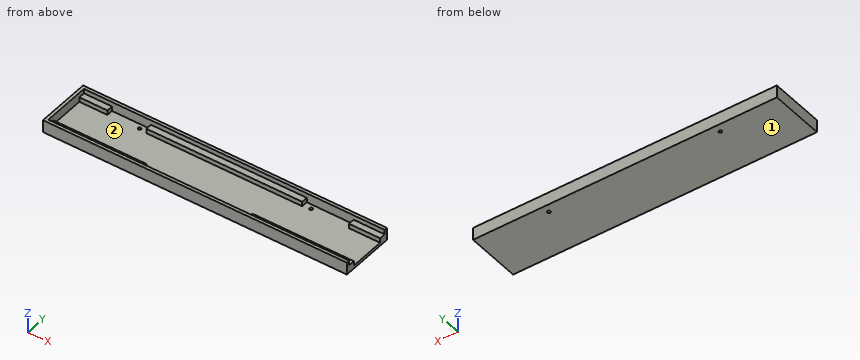
```python
from build123d import *

# Parameters (mm, degrees)
F0_W      = 195
F0_H      = 35
F1_DEPTH  = 2
F2_W      = 195
F2_H      = 2
F3_DEPTH  = 6
F4_W      = 18
F4_H      = 4
F5_DEPTH  = 3
F6_W      = 100
F6_H      = 4
F7_DEPTH  = 3
F8_W      = 20
F8_H      = 4
F9_DEPTH  = 3
F10_W     = 2
F10_H     = 31
F11_DEPTH = 6
F12_W     = 15
F12_H     = 2
F13_DEPTH = 3
F14_W     = 60
F14_H     = 2
F15_DEPTH = 3
F17_D     = 2


with BuildPart() as f1:
    # F0 (on Top) → F1 (new body)
    with BuildSketch(Plane.XY):
        Rectangle(F0_W, F0_H)
    extrude(amount=F1_DEPTH)

    # F2 (on face) → F3 (join)
    with BuildSketch(Plane.XY.offset(2)):
        with Locations((0, -16.5)):
            Rectangle(F2_W, F2_H)
        with Locations((0, 16.5)):
            Rectangle(F2_W, F2_H)
    extrude(amount=F3_DEPTH)

    # F4 (on face) → F5 (join)
    with BuildSketch(Plane.XY.offset(2)):
        with Locations((-86.5, 13.5)):
            Rectangle(F4_W, F4_H)
    extrude(amount=F5_DEPTH)

    # F6 (on face) → F7 (join)
    with BuildSketch(Plane.XY.offset(2)):
        with Locations((-2.5, 13.5)):
            Rectangle(F6_W, F6_H)
    extrude(amount=F7_DEPTH)

    # F8 (on face) → F9 (join)
    with BuildSketch(Plane.XY.offset(2)):
        with Locations((87.5, 13.5)):
            Rectangle(F8_W, F8_H)
    extrude(amount=F9_DEPTH)

    # F10 (on face) → F11 (join)
    with BuildSketch(Plane.XY.offset(2)):
        with Locations((-96.5, 0)):
            Rectangle(F10_W, F10_H)
    extrude(amount=F11_DEPTH)

    # F12 (on face) → F13 (join)
    with BuildSketch(Plane.XY.offset(2)):
        with Locations((90, -14.5)):
            Rectangle(F12_W, F12_H)
        Polygon((82.5, -13.5), (97.5, -13.5), (97.5, -11.5), (32.5, -11.5), (32.5, -13.5), align=None)
    extrude(amount=F13_DEPTH)

    # F14 (on face) → F15 (join)
    with BuildSketch(Plane.XY.offset(2)):
        with Locations((-65.5, -12.5)):
            Rectangle(F14_W, F14_H)
    extrude(amount=F15_DEPTH)

    # F17 (through all)
    with Locations(Plane.XY.offset(2)):
        with Locations((-57.5, 12.5), (52.5, 12.5)):
            Hole(F17_D / 2)


solid = f1.part
```
Input: part model. Units: mm. Frame: model coordinates. Face numbers are marked on the shaded views. Coordinates: 2 decimals unless noted, no trailing zeros. Write each loop counter-clockwise with the first axis right and the second up, starting at its lowest first coordinate (ties: lowest second). Pieces come first, ordered by that corner, then holes. Notation, with made-up numbers: (-16.75, -9.75) -> (23.25, -9.75) arc R27 ccw to (23.25, 29.25) -> close; hole circle Ø3 at (33.5, -36.5). An arc over 180 degrees is marked (long way). Answer as a JSON object with one key per item and string values.
1. First-contact query: P1, Ø2, axis at x = 23.5, y = -0.5, coming from the +Z side; P2, Ø1.6, axis at x = -57.5, y = 12.5, coming from the -Z side; P3, Ø2, axis at x = 16.5, y = 13, coming from the +Z side. Flat tips, straight axial feed; report the tip coordinate or a pass-through.
Result set:
{"P1": "stops at z = 2", "P2": "passes through", "P3": "stops at z = 5"}
2. Section B-B on y = 6. Return the cut outline in (x, z).
Result set:
{"outline": "(-97.5, 0) -> (97.5, 0) -> (97.5, 2) -> (-95.5, 2) -> (-95.5, 8) -> (-97.5, 8) -> close"}
3. Section A-A on x = -70.5. Return the cut outline in (y, z), then the cut area to 3 significant figures.
Result set:
{"outline": "(-17.5, 0) -> (17.5, 0) -> (17.5, 8) -> (15.5, 8) -> (15.5, 2) -> (-11.5, 2) -> (-11.5, 5) -> (-13.5, 5) -> (-13.5, 2) -> (-15.5, 2) -> (-15.5, 8) -> (-17.5, 8) -> close", "area": "100 mm2"}
4. Mould query, pull axis Y, two halves, no side actions, for the marked faces 1 and 2. Classes: released by +Y, released by -Y, zero draft, split by the parting line, or undercut.
Result set:
{"face 1": "zero draft", "face 2": "undercut"}
5. Section C-C on x = 34.5. Return the cut outline in (y, z).
Result set:
{"outline": "(-17.5, 0) -> (17.5, 0) -> (17.5, 8) -> (15.5, 8) -> (15.5, 5) -> (11.5, 5) -> (11.5, 2) -> (-11.5, 2) -> (-11.5, 5) -> (-13.5, 5) -> (-13.5, 2) -> (-15.5, 2) -> (-15.5, 8) -> (-17.5, 8) -> close"}
6. Material intervals for line 1 (Y direction, x = -58, z = 2.75); line 2 (Y direction, x = -84.5, z = 7.5); line 3 (Y direction, x = 35.5, z = 3), sorted ascending. Write a range as from..to.
Result set:
{"line 1": "y = -17.5..-15.5, -13.5..-11.5, 15.5..17.5", "line 2": "y = -17.5..-15.5, 15.5..17.5", "line 3": "y = -17.5..-15.5, -13.5..-11.5, 11.5..17.5"}
